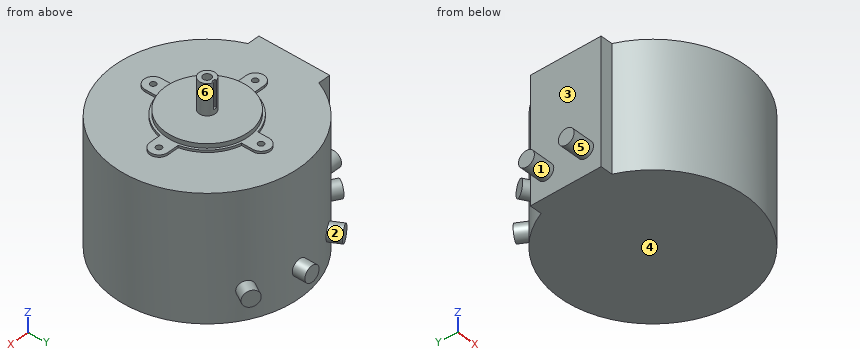
```python
from build123d import *

# Parameters (mm, degrees)
SZKIC1_R                    = 128
DODANIE_WYCI_GNI_CIE1_DEPTH = 172
SZKIC2_W                    = 135
SZKIC2_H                    = 98
DODANIE_WYCI_GNI_CIE2_DEPTH = 172
SZKIC3_R                    = 11
DODANIE_WYCI_GNI_CIE3_DEPTH = 30
SZKIC5_W                    = 11
SZKIC5_H                    = 25
SZYK_START                  = -145
SZYK_KO_OWY1_OUTLINE_R      = 11
SZYK_KO_OWY1_DEPTH          = 17.473532259
SZYK_KO_OWY1_2_OUTLINE_R    = 11
SZYK_KO_OWY1_2_DEPTH        = 17.473532259
SZYK_START_2                = 127.526467741
SZYK_KO_OWY1_3_OUTLINE_R    = 11
SZYK_KO_OWY1_3_DEPTH        = 17.473532259
SZKIC6_R                    = 57.15
DODANIE_WYCI_GNI_CIE4_DEPTH = 9.2
SZKIC7_R                    = 11.115
DODANIE_WYCI_GNI_CIE5_DEPTH = 42.6
SZKIC8_W                    = 4.78
SZKIC8_H                    = 5
WYTNIJ_WYCI_GNI_CIE1_DEPTH  = 36
SZKIC9_R                    = 5.556
WYTNIJ_WYCI_GNI_CIE2_DEPTH  = 30
DODANIE_WYCI_GNI_CIE6_DEPTH = 3.2
SZKIC11_R                   = 3.97
WYTNIJ_WYCI_GNI_CIE3_DEPTH  = 19
SZYK_KO_OWY2_COUNT          = 4
SZKIC12_R                   = 60.15
DODANIE_WYCI_GNI_CIE7_DEPTH = 3.2


# Read off the part's stored shape, not the designer's step: Szyk kołowy1
with BuildPart() as part:
    # Szkic1 → Dodanie-wyciągnięcie1 (new body)
    with BuildSketch(Plane.XY):
        Circle(SZKIC1_R)
    extrude(amount=DODANIE_WYCI_GNI_CIE1_DEPTH)

    # Szkic2 → Dodanie-wyciągnięcie2 (add)
    with BuildSketch(Plane.XY.offset(172)):
        with Locations((-67.5, 0)):
            Rectangle(SZKIC2_W, SZKIC2_H)
    extrude(amount=-DODANIE_WYCI_GNI_CIE2_DEPTH)

    # Szkic3 → Dodanie-wyciągnięcie3 (add)
    with BuildSketch(Plane.ZY.offset(135)):
        with Locations((33, 27.5)):
            Circle(SZKIC3_R)
        with Locations((33, -27.5)):
            Circle(SZKIC3_R)
    extrude(amount=DODANIE_WYCI_GNI_CIE3_DEPTH)

    # Szkic5 → Obrót1 (revolve)
    with BuildSketch(Plane(origin=(0, 0, 41), x_dir=(-1, 0, 0), z_dir=(0, 0, -1)), mode=Mode.PRIVATE) as obr_t1_sk:
        with Locations((-5.5, 132.5)):
            Rectangle(SZKIC5_W, SZKIC5_H)
    revolve(obr_t1_sk.sketch.rotate(Axis((0, 145, 41), (0, -1, 0)), 180), axis=Axis((0, 145, 41), (0, -1, 0)))

    # Szyk kołowy1 outline → Szyk kołowy1 (add)
    with BuildSketch(Plane(origin=(0, 0, 0), x_dir=(0.866025403784438, 0.500000000000001, 0), z_dir=(0.500000000000001, -0.866025403784438, 0)).offset(SZYK_START)):
        with Locations((0, 41)):
            Circle(SZYK_KO_OWY1_OUTLINE_R)
    extrude(amount=SZYK_KO_OWY1_DEPTH)

    # Szyk ko_owy1 2 outline → Szyk ko_owy1 2 (add)
    with BuildSketch(Plane(origin=(0, 0, 0), x_dir=(0.49999999999999767, 0.86602540378444, 0), z_dir=(0.8660254037844399, -0.49999999999999795, 0)).offset(SZYK_START)):
        with Locations((0, 41)):
            Circle(SZYK_KO_OWY1_2_OUTLINE_R)
    extrude(amount=SZYK_KO_OWY1_2_DEPTH)

    # Szyk ko_owy1 3 outline → Szyk ko_owy1 3 (add)
    with BuildSketch(Plane(origin=(0, 0, 0), x_dir=(0.866025403784438, -0.500000000000001, 0), z_dir=(0.500000000000001, 0.866025403784438, 0)).offset(SZYK_START_2)):
        with Locations((0, -41)):
            Circle(SZYK_KO_OWY1_3_OUTLINE_R)
    extrude(amount=SZYK_KO_OWY1_3_DEPTH)

    # Szkic6 → Dodanie-wyciągnięcie4 (add)
    with BuildSketch(Plane.XY.offset(172)):
        Circle(SZKIC6_R)
    extrude(amount=DODANIE_WYCI_GNI_CIE4_DEPTH)

    # Szkic7 → Dodanie-wyciągnięcie5 (add)
    with BuildSketch(Plane.XY.offset(181.2)):
        Circle(SZKIC7_R)
    extrude(amount=DODANIE_WYCI_GNI_CIE5_DEPTH)

    # Szkic8 → Wytnij-wyciągnięcie1 (cut)
    with BuildSketch(Plane.XY.offset(223.8)):
        with Locations((0, 10.965)):
            Rectangle(SZKIC8_W, SZKIC8_H)
    extrude(amount=-WYTNIJ_WYCI_GNI_CIE1_DEPTH, mode=Mode.SUBTRACT)

    # Szkic9 → Wytnij-wyciągnięcie2 (cut)
    with BuildSketch(Plane.XY.offset(223.8)):
        Circle(SZKIC9_R)
    extrude(amount=-WYTNIJ_WYCI_GNI_CIE2_DEPTH, mode=Mode.SUBTRACT)

    # Szkic10 → Dodanie-wyciągnięcie6 (add)
    with BuildSketch(Plane.XY.offset(172)):
        with BuildLine():
            Line((-73.545292167, 12.5), (-74.6, 12.5))
            ThreePointArc((-74.6, 12.5), (-87.1, 0), (-74.6, -12.5))
            Line((-74.6, -12.5), (-73.545292167, -12.5))
            Line((-73.545292167, -12.5), (-55.766230821, -12.5))
            ThreePointArc((-55.766230821, -12.5), (-57.15, 0), (-55.766230821, 12.5))
            Line((-55.766230821, 12.5), (-73.545292167, 12.5))
        make_face()
    dodanie_wyci_gni_cie6 = extrude(amount=DODANIE_WYCI_GNI_CIE6_DEPTH)

    # Szkic11 → Wytnij-wyciągnięcie3 (cut)
    with BuildSketch(Plane.XY.offset(175.2)):
        with Locations((-74.6, 0)):
            Circle(SZKIC11_R)
    wytnij_wyci_gni_cie3 = extrude(amount=-WYTNIJ_WYCI_GNI_CIE3_DEPTH, mode=Mode.SUBTRACT)

    # Szyk kołowy2: Dodanie-wyciągnięcie6, Wytnij-wyciągnięcie3 ×4 about axis
    szyk_ko_owy2_axis = Axis((0, 0, 0), (0, 0, 1))
    add([dodanie_wyci_gni_cie6.rotate(szyk_ko_owy2_axis, i * 360 / SZYK_KO_OWY2_COUNT) for i in range(1, SZYK_KO_OWY2_COUNT)])
    add([wytnij_wyci_gni_cie3.rotate(szyk_ko_owy2_axis, i * 360 / SZYK_KO_OWY2_COUNT) for i in range(1, SZYK_KO_OWY2_COUNT)], mode=Mode.SUBTRACT)

    # Szkic12 → Dodanie-wyciągnięcie7 (add)
    with BuildSketch(Plane.XY.offset(172)):
        Circle(SZKIC12_R)
    extrude(amount=DODANIE_WYCI_GNI_CIE7_DEPTH)


solid = part.part
```
Here's how the part is built. I have some questions about the finished solid (model axes, mm). Face numbers are marked on the shaded views. A direction names the side the tool comes from. Give positions to 0.01 mm unless a question says otherwise; leave off trailing zeros. Write each loop counter-clockwise with the first axis right and the second up, starting at its lowest first coordinate (ties: lowest second). Pieces come first, ordered by that corner, then holes. Notation, with made-up numbers: (58.25, 24) -> (69.25, 24) arc R22 ccw to (69.25, 41) -> close; hole circle Ø5 at (81, -0.75). An arc over 180 degrees is marked (long way). Write each question's results on one line, items separated by ' | '.
Item 1: We'd pull the mould along X, two halves only. Please class the marked faces 1, 2 and 3: pulls with the +X half, pulls with the -X half, needs draft (parallel to the pull), parting line crosses it, or undercut.
Output:
face 1: needs draft | face 2: undercut | face 3: pulls with the -X half
Item 2: Suppose I cut it at B-B on z = 89. Write out the boundary of the cut face in (x, y), plus the area to 3 significant figures.
Output:
outline: (-135, -49) -> (-118.25, -49) arc R128 ccw (long way) to (-118.25, 49) -> (-135, 49) -> close | area: 52,500 mm^2
Item 3: Suppose I cut it at D-D on y = -27.5. Write out the boundary of the cut face in (x, z).
Output:
outline: (-165, 22) -> (-135, 22) -> (-135, 0) -> (125.01, 0) -> (125.01, 172) -> (53.5, 172) -> (53.5, 175.2) -> (50.1, 175.2) -> (50.1, 181.2) -> (-50.1, 181.2) -> (-50.1, 175.2) -> (-53.5, 175.2) -> (-53.5, 172) -> (-135, 172) -> (-135, 44) -> (-165, 44) -> close
Item 4: Suppose I cut it at C-C on x = -18. Write out the boundary of the cut face in (y, z).
Output:
outline: (-126.73, 0) -> (126.73, 0) -> (126.73, 172) -> (57.39, 172) -> (57.39, 175.2) -> (54.24, 175.2) -> (54.24, 181.2) -> (-54.24, 181.2) -> (-54.24, 175.2) -> (-57.39, 175.2) -> (-57.39, 172) -> (-126.73, 172) -> close
Item 5: Suppose I cut it at A-A on y = 0. Write out the boundary of the cut face in (x, z) (3 decimals), plus the area to 3 significant figures.
Output:
outline: (-135, 0) -> (128, 0) -> (128, 172) -> (87.1, 172) -> (87.1, 175.2) -> (78.57, 175.2) -> (78.57, 156.2) -> (70.63, 156.2) -> (70.63, 175.2) -> (57.15, 175.2) -> (57.15, 181.2) -> (11.115, 181.2) -> (11.115, 223.8) -> (5.556, 223.8) -> (5.556, 193.8) -> (-5.556, 193.8) -> (-5.556, 223.8) -> (-11.115, 223.8) -> (-11.115, 181.2) -> (-57.15, 181.2) -> (-57.15, 175.2) -> (-70.63, 175.2) -> (-70.63, 156.2) -> (-78.57, 156.2) -> (-78.57, 175.2) -> (-87.1, 175.2) -> (-87.1, 172) -> (-135, 172) -> close | area: 46,800 mm^2
Item 6: On a 3-axis mill with a long thin cutter (end or side, diameter ignored), from which of +Z, -Z, +X, -X, +Y, -Y can I reach the whole of each face in a straight line? I mean the marked faces 4, 5 and 6. Say none if no direction works.
Output:
face 4: -Z, +X, -X, +Y, -Y | face 5: -X | face 6: +Z
Item 7: For pin 1 Ø18 at (x, y) = (0, 0) entering from -Z; pin 2 Ø7 at (x, y) = (0, -74.6) entering from +Z; pin 3 Ø8 at (y, z) = (8.5, 170.5) entering from +X; pin 4 Ø2.5 at (y, z) = (69.5, 173) entering from +X, each with a flat end and sliding along its axis, tell me the tip position at first contact or that it passes through.
Output:
pin 1: stops at z = 0 | pin 2: stops at z = 156.2 | pin 3: stops at x = 127.92 | pin 4: stops at x = 107.97
Item 8: If I drill on L1, parallel to Z at x = 56.5, y = 96; L2, parallel to Y at x = 0, z = 208 (3 decimals); L3, parallel to Y at x = -128, z = 164.5, over which ranges is the centre line in solid material (lowest first)?
Output:
L1: z = 0 to 172 | L2: y = -11.115 to -5.556, 5.556 to 8.465 | L3: y = -49 to 49
